For this review, take the finished solid that the model builds, in its own axes (mm). Face numbers are marked on the shaded views. A direction names the side the tool comes from. Round coordinates to 2 decimals unless told otherwise and drop trailing zeros. Write each loop counter-clockwise with the first axis right and the second up, starting at its lowest first coordinate (ties: lowest second). Pieces come first, ordered by that corner, then holes. Notation, with made-up numbers: (20.25, 86) - (33.25, 86) arc R25 cw to (33.25, 100) - close; hole circle Ø3 at (-9, -24). An arc over 180 degrees is marked (long way). One line per item, written item: value. Start each with the question number.
Q1. Mouldability with a two-part tool opening along Y and no side actions: class the marked faces 1, 2 and 3 as +Y half, -Y half, draft (parallel to the pull), parting line (faces both ways), or undercut.
Q2. Clearance check with flat-ended pins moving along their axes: pin 1 Ø2 at (y, z) = (0.5, 1) entering from +X; pin 2 Ø1.5 at (x, y) = (2, -0.5) entering from -Z; pin 3 Ø1.5 at (x, z) = (6.5, -1.5) entering from +Y; pin 4 Ø1 at (x, z) = (1.5, -0.5) entering from -Y. State where each tip first meets the part, or that it passes through.
Q3. Add section A-A on x = 3.5. Write out the cut boundary in (y, z).
Q4. Tool access review of the marked faces 4, 5 and 6: name each direction out of +Z, -Z, +X, -X, +Y, -Y from which nothing blocks a thin tool from reaching the whole face with its end or side.
Q5. Add section B-B on z = -1.75. Write out the cut boundary in (x, y), and give its area (3 significant figures).
Q6. For probe 1 along Y at (x, z) = (-0.75, 0.1); probe 2 along X at (y, z) = (0.4, 1.5); probe 3 along Y at (x, z) = (9.5, -0.75), list the stretches that pass through material, from the lowest coordinate up.
Autodesk Inventor part; units mm, degrees
ref_plane "Work Plane1" through (29, 0, 0) normal (0, -1, 0) x (1, 0, 0)
ref_plane "YZ Plane" through (0, 0, 0) normal (1, 0, 0) x (0, 1, 0)
ref_plane "XZ Plane" through (0, 0, 0) normal (0, 1, 0) x (-1, 0, 0)
sketch "Sketch1" plane through (0, 0, 0) normal (0, 0, 1) x (1, 0, 0)
  line L0 (0.2067, 0) -> (10, 0)
  line L1 (10, 0) -> (10, 1.25)
  line L2 (10, 1.25) -> (1.5, 1.25)
  line L3 (1.5, 1.25) -> (1.1932, 1.25)
  line L4 (1.1932, 1.25) -> (0, 1.25)
  line L5 (0, 1.25) -> (0, 2.2)
  line L6 (0, 2.2) -> (-1.5, 2.2)
  line L7 (-1.5, 2.2) -> (-1.5, 1.1547)
  line L8 (-1.5, 1.1547) -> (-0.46, 1.1547)
  line L9 (-0.46, 1.1547) -> (0.2067, 0)
  line L10 (-3.8, 0) -> (12.3, 0)
  line L11 (0, -0.44) -> (0, 2.64)
  line L12 (1.5, 1.25) -> (0, 1.25) construction
  dimension "d1" = 8.5
  dimension "d2" = 0.3068
  dimension "d3" = 1.5
  dimension "d4" = 1.04
  dimension "d5" = 60
  dimension "d6" = 2.5
  dimension "d7" = 2.5
  dimension "d8" = 2.3094
  dimension "d9" = 4.4
  dimension "d26" = 10
revolve "Body" add sketch "Sketch1" angle 360 about axis through (0.2067, 0, 0) along (1, 0, 0) contours L9 L11 L4 L3 L2 L1 L0 | L9 L8 L7 L6 L5 L11
sketch "Sketch2" plane through (-1.5, 0, 0) normal (-1, 0, 0) x (0, 0, 1)
  circle A0 centre (0, 0) radius 1.1547
  line L0 (0, -3.08) -> (0, 3.08)
  line L1 (-3.08, 0) -> (3.08, 0)
  line L2 (1.1547, 0) -> (0.5774, -1)
  line L3 (0.5774, -1) -> (-0.5774, -1)
  line L4 (-0.5774, -1) -> (-1.1547, 0)
  line L5 (-1.1547, 0) -> (-0.5774, 1)
  line L6 (-0.5774, 1) -> (0.5774, 1)
  line L7 (0.5774, 1) -> (1.1547, 0)
extrude "Slot" add sketch "Sketch2" against normal up to next contours L7 A0 | A0 L2 | L6 L0 A0 | A0 L0 L3 | L0 L6 A0 | A0 L3 L0 | L4 A0 | A0 L5
thread "Thread"
chamfer "Chamfer1" distance 0.3067 distance2 0.3067 1 edges at (10, -1.25, 0) measured on face at (10, -0.2714, -0.6096)
ref_plane "Work Plane1" through (29, 0, 0) normal (0, -1, 0) x (1, 0, 0)
fillet "Fillet2" radius 0.3 1 edges at (0, -1.25, 0)
equation "\"d30\" = R"
equation "\"d13\" = GEL"
equation "\"d15\" = -0.5 * SPD + 0.5 * GD"
equation "\"d16\" = GUL"
equation "\"d1\" = GEL"
equation "\"d4\" = INTI"
equation "\"d8\" = 1.1547 * SW"
equation "\"d26\" = NLG"
equation "\"GD\" = NND"
equation "\"NLG\" = 10"
equation "\"GEL\" = 8.5"
equation "\"KOD\" = 5.7"
equation "\"KOH\" = 1.65"
equation "\"INTI\" = 1.04"
equation "\"GAL\" = 0.61345 * PTC"
equation "\"GUL\" = 0.61345 * PTC"
equation "\"BDM\" = NND"
equation "\"SW\" = 2"
equation "\"RR\" = 1.45"
equation "\"SPD\" = NND - 1.2269 * PTC"
equation "\"R\" = 0.3"
equation "\"TOA\" = 30deg"
equation "\"GD1\" = THREADDIA - 1.2269 * PTC"
equation "\"THREADDIA\" = 3"
equation "\"PTC\" = 0.5"
equation "\"NND\" = 3"
equation "\"KOH1\" = 0.2"
equation "\"E0\" = 2.303"
properties part number "ISO 7380-1 - M3 x 10" material "Steel"
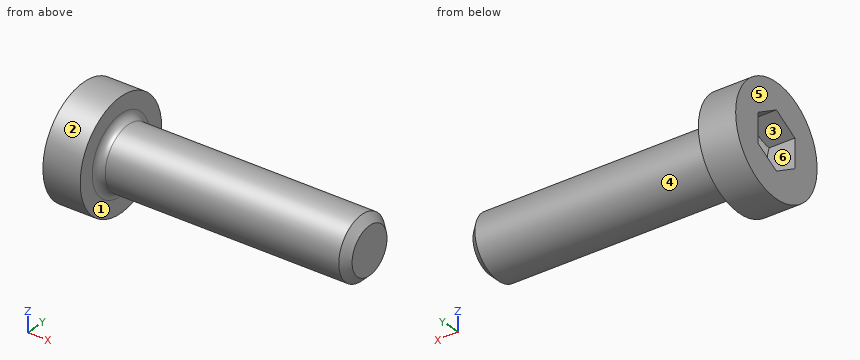
Result set:
1. face 1: draft
1. face 2: parting line
1. face 3: undercut
2. pin 1: stops at x = 10
2. pin 2: stops at z = -1.25
2. pin 3: stops at y = 1
2. pin 4: stops at y = -1.25
3. outline: circle Ø2.5 at (0, 0)
4. face 4: +X
4. face 5: +Z, -Z, -X, +Y, -Y
4. face 6: -X
5. outline: (-1.5, -1.33) - (0, -1.33) - (0, 1.33) - (-1.5, 1.33) - close
5. area: 4.00 mm^2
6. probe 1: y = -2.2 to -1, 1 to 2.2
6. probe 2: x = -1.5 to 0
6. probe 3: y = -1 to 1
